Could you check a few things on this model? Use its own coordinates, in mm. Give positions to 0.01 mm unless a question says otherwise; leave off trailing zeros. Order: outer loops, then holes, each group sorted by start corner. A loop starts at its lowest first (then second) coordinate and runs counter-clockwise, first axis right, second up. Notation, with made-up numbers: (32, 62) - (42, 62) arc R19 cw to (42, 95) - close; hole circle Ø10 at (53, -24.75). An arc over 180 degrees is marked (long way). Put each result on its own line as item: value.
Autodesk Inventor part; units mm, degrees
ref_plane "YZ Plane" through (0, 0, 0) normal (1, 0, 0) x (0, 1, 0)
ref_plane "XZ Plane" through (0, 0, 0) normal (0, 1, 0) x (-1, 0, 0)
ref_plane "XY Plane" through (0, 0, 0) normal (0, 0, 1) x (1, 0, 0)
sketch "スケッチ1" plane through (0, 0, 0) normal (0, 0, 1) x (1, 0, 0)
  circle A0 centre (0, 0) radius 70
  circle A1 centre (0, 0) radius 57
  dimension "d0" = 140
  dimension "d1" = 114
extrude "押し出し1" add sketch "スケッチ1" along normal blind 8.2
sketch "スケッチ2" plane through (0, 0, 8.2) normal (0, 0, 1) x (1, 0, 0)
  point P0 (0, 0)
  point P1 (-64, 0)
  point P2 (0, -64)
  point P3 (64, 0)
  point P4 (0, 64)
  dimension "d4" = 64
  dimension "d7" = 360
hole "穴1" at (-64, 0, 8.2) at (0, -64, 8.2) at (64, 0, 8.2) at (0, 64, 8.2) direction (0, 0, -1) diameter 4.4 end through all countersink diameter 10 countersink angle 90
fillet "フィレット1" radius 0.5 4 edges at (-70, 0, 0) (-57, 0, 0) (-70, 0, 8.2) (-57, 0, 8.2)
properties part number "TurnTable_140_Outer" material "鋼、合金"
1) We'd pull the mould along X, two halves only. Please class faces 1 (the conical face through (65.61, 1.75, 5.58)), 2 (the conical face through (-61.645, 0.309, 5.575)), 3 (the cylindrical face through (-55.55, 42.594, 4.05)), 4 (the flat face through (-57, 11, 8.2)): pulls with the +X half, pulls with the -X half, needs draft (parallel to the pull), parting line crosses it, or undercut.
Filled in:
face 1: undercut
face 2: undercut
face 3: parting line crosses it
face 4: needs draft
2) If I drill on line 1 (Y direction, x = 0, z = 4.25); line 2 (Y direction, x = 0, z = 6); line 3 (Y direction, x = -43, z = 1), over which ranges is the centre line in solid material (lowest first)? Write a range as [from, to].
Filled in:
line 1: y = [-70, -66.2], [-61.8, -57], [57, 61.8], [66.2, 70]
line 2: y = [-70, -66.8], [-61.2, -57], [57, 61.2], [66.8, 70]
line 3: y = [-55.24, -37.42], [37.42, 55.24]
3) Suppose I cut it at A-A, the plane y = 0. List the corners of the cut face in (x, z) for me.
Filled in:
outline: (-70, 0.5) arc R0.5 ccw to (-69.5, 0) - (-66.2, 0) - (-66.2, 5.4) - (-69, 8.2) - (-69.5, 8.2) arc R0.5 ccw to (-70, 7.7) - close; (-61.8, 0) - (-57.5, 0) arc R0.5 ccw to (-57, 0.5) - (-57, 7.7) arc R0.5 ccw to (-57.5, 8.2) - (-59, 8.2) - (-61.8, 5.4) - close; (57, 0.5) arc R0.5 ccw to (57.5, 0) - (61.8, 0) - (61.8, 5.4) - (59, 8.2) - (57.5, 8.2) arc R0.5 ccw to (57, 7.7) - close; (66.2, 0) - (69.5, 0) arc R0.5 ccw to (70, 0.5) - (70, 7.7) arc R0.5 ccw to (69.5, 8.2) - (69, 8.2) - (66.2, 5.4) - close
4) Suppose I cut it at C-C, the plane z = 4. List the corners of the cut face in (x, y) for me.
Filled in:
outline: circle Ø140 at (0, 0); hole circle Ø4.4 at (-64, 0); hole circle Ø114 at (0, 0); hole circle Ø4.4 at (0, -64); hole circle Ø4.4 at (0, 64); hole circle Ø4.4 at (64, 0)
5) I'm going to push flat-ended pins straight in: pin 1 (1.5 mm diameter, centred on y = 19.5, z = 5.5, fed in from +X); pin 2 (4 mm diameter, centred on x = -40.5, y = 36, fed in from +Z); pin 3 (5 mm diameter, centred on x = -64, y = 0, fed in from +Z). Where does each tip first touch, or does it pass through?
Filled in:
pin 1: stops at x = 67.44
pin 2: passes through
pin 3: stops at z = 5.7
